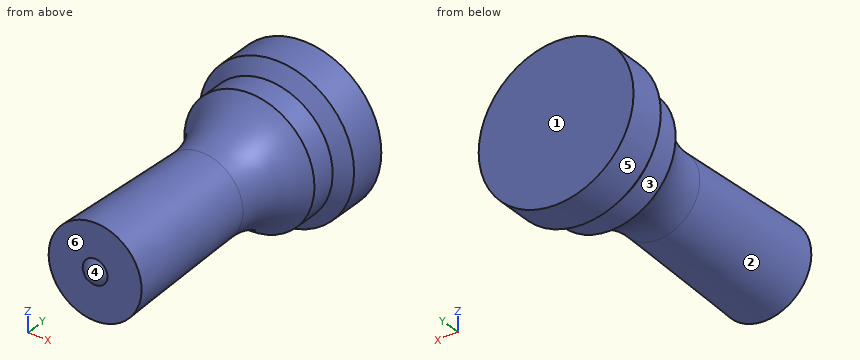
from build123d import *


with BuildPart() as part:
    # Sketch1 → Revolve1 (revolve)
    with BuildSketch(Plane.XY, mode=Mode.PRIVATE) as revolve1_sk:
        with BuildLine():
            Line((0, 48), (12.5, 48))
            Line((12.5, 48), (12.5, 42))
            Line((12.5, 42), (10.5, 40))
            Line((10.5, 40), (10.5, 36))
            ThreePointArc((10.5, 36), (7.569816074, 31.103274793), (6.680531261, 25.466514365))
            Line((6.680531261, 25.466514365), (7.5, 2))
            Line((7.5, 2), (2, 2))
            Line((2, 2), (0, 0))
            Line((0, 0), (0, 48))
        make_face()
    revolve(revolve1_sk.sketch.rotate(Axis((0, 0, 0), (0, 1, 0)), 90), axis=Axis((0, 0, 0), (0, 1, 0)))  # turned: the seam where the file's is


solid = part.part
Source: CAD feature listing. Evaluate the final solid. Frame: model axes, mm. Face numbers are marked on the shaded views. A direction names the side the tool comes from. Round coordinates to 2 decimals unless told otherwise and drop trailing zeros. Write each loop counter-clockwise with the first axis right and the second up, starting at its lowest first coordinate (ties: lowest second). Pieces come first, ordered by that corner, then holes. Notation, with made-up numbers: M 33.25,9 L 60.25,9 A32 cw 60.25,39 Z; hole C 32.5,65.5 d3. An arc over 180 degrees is marked long. One line per item, written item: value. Start each with the question number.
Item 1: Ray query, L1, parallel to Y at x = -1, z = -6; L2, parallel to X at y = 29.5, z = -4.75; L3, parallel to Y at x = -1.75, z = 9.75. Return the intervals inside material, ascending. Write a range as from..to.
Item 2: Section query A-A (y = 39). Return the cut outline in (x, z), plus the area to 3 significant figures.
Item 3: Mould query, pull axis Y, two halves, no side actions, for the marked faces 1, 2, 3 and 4. Classes: pulls with the +Y half, pulls with the -Y half, needs draft (parallel to the pull), parting line crosses it, or undercut.
Item 4: Set-up query: the marked faces 5 and 6. Return all of +Z, -Z, +X, -X, +Y, -Y with unobstructed straight access to the full face (end or side cutting, diameter ignored); none if empty.
Item 5: Section query B-B (y = 7.5). Return the cut outline in (x, z), plus the area to 3 significant figures.
Item 6: Pin query (flat end, axial travel): pin 1 (10 mm diameter, centred on x = 1.5, y = 31.5, fed in from +Z); pin 2 (12 mm diameter, centred on x = 2.5, z = -0.5, fed in from -Y); pin 3 (4 mm diameter, centred on x = -6, y = 13.5, fed in from -Z); pin 4 (12 mm diameter, centred on x = -5.5, y = 30, fed in from +Z). Return the tip coordinate at first contact, or that it passes through.
Result set:
1. L1: y = 2..48
1. L2: x = -5.26..5.26
1. L3: y = 35.29..48
2. outline: C 0,0 d21
2. area: 346 mm²
3. face 1: pulls with the +Y half
3. face 2: undercut
3. face 3: needs draft
3. face 4: pulls with the -Y half
4. face 5: +Y, -Y
4. face 6: -Y
5. outline: C 0,0 d14.62
5. area: 168 mm²
6. pin 1: stops at z = 10.5
6. pin 2: stops at y = 0
6. pin 3: stops at z = -5.87
6. pin 4: stops at z = 9.59
